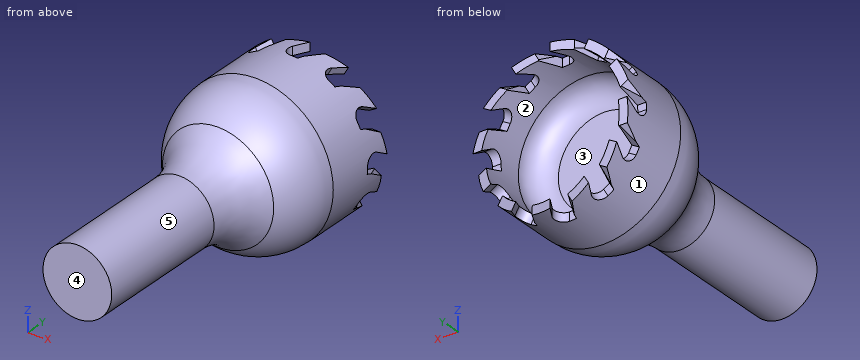
```python
from build123d import *

# Parameters (mm, degrees)
CUT_EXTRUDE1_DEPTH = 19.304
CIRPATTERN2_COUNT  = 12


with BuildPart() as part:
    # Sketch1 → Revolve1 (revolve)
    with BuildSketch(Plane.XY, mode=Mode.PRIVATE) as revolve1_sk:
        with BuildLine():
            Line((0, 0), (-4.7625, 0))
            Line((-4.7625, 0), (-4.7625, 19.05))
            ThreePointArc((-4.7625, 19.05), (-5.529894723, 22.907953795), (-7.71525, 26.178569096))
            ThreePointArc((-7.71525, 26.178569096), (-9.900605277, 29.449184398), (-10.668, 33.307138193))
            Line((-10.668, 33.307138193), (-10.668, 43.307138193))
            Line((-10.668, 43.307138193), (-9.468, 43.307138193))
            Line((-9.468, 43.307138193), (-9.468, 36.482138193))
            ThreePointArc((-9.468, 36.482138193), (-8.53806403, 34.237074162), (-6.293, 33.307138193))
            Line((-6.293, 33.307138193), (0, 33.307138193))
            Line((0, 33.307138193), (0, 0))
        make_face()
    revolve(revolve1_sk.sketch.rotate(Axis((0, 33.307138193, 0), (0, -1, 0)), 270), axis=Axis((0, 33.307138193, 0), (0, -1, 0)))

    # Sketch2 → Cut-Extrude1 (cut)
    with BuildSketch(Plane.XY):
        with BuildLine():
            Line((0, 43.307138193), (1.04608221, 41.495270656))
            ThreePointArc((1.04608221, 41.495270656), (1.04608221, 40.287358966), (0, 39.68340312))
            Line((0, 39.68340312), (-0.966946132, 39.68340312))
            Line((-0.966946132, 39.68340312), (-2.440808814, 43.792749848))
            Line((-2.440808814, 43.792749848), (4.66649361, 43.792749848))
            Line((4.66649361, 43.792749848), (4.66649361, 39.68340312))
            Line((4.66649361, 39.68340312), (2.934442802, 42.68340312))
            Line((2.934442802, 42.68340312), (0, 43.307138193))
        make_face()
    cut_extrude1 = extrude(amount=-CUT_EXTRUDE1_DEPTH, mode=Mode.SUBTRACT)

    # CirPattern2: Cut-Extrude1 ×12 about axis
    cirpattern2_axis = Axis((0, 0, 0), (0, 1, 0))
    for i in range(1, CIRPATTERN2_COUNT):
        add(cut_extrude1.rotate(cirpattern2_axis, i * 360 / CIRPATTERN2_COUNT), mode=Mode.SUBTRACT)


solid = part.part
```
The model under review builds one solid part; all positions refer to its coordinate system, in mm. Face numbers are marked on the shaded views. A direction names the side the tool comes from. Round coordinates to 2 decimals unless told otherwise and drop trailing zeros. Order: outer loops, then holes, each group sorted by start corner. A loop starts at its lowest first (then second) coordinate and runs counter-clockwise, first axis right, second up. Notation, with made-up numbers: (-2.75, 14.25) - (51.25, 14.25) arc R15 ccw to (51.25, 27.25) - close; hole circle Ø2 at (-32.5, 55.25). An arc over 180 degrees is marked (long way). Answer in a Markdown table with one row per item.
(1) Clearance check with flat-ended pins moving along their axes: P1, Ø12, axis at y = 27.5, z = 8, coming from the -X side; P2, Ø1, axis at x = 4.5, z = -8, coming from the -Y side; P3, Ø1.5, axis at x = 5.5, y = 22.5, coming from the +Z side. State where each tip first meets the part, or that it passes through.
Result set:
| item | result |
|---|---|
| P1 | stops at x = -9.92 |
| P2 | stops at y = 27.29 |
| P3 | stops at z = 2.63 |
(2) For line 1 (X direction, y = 39.5, z = 0); line 2 (X direction, y = 18, z = -0.25); line 3 (X direction, y = 36.5, z = 7.75), list the stretches that pass through material, from the lowest coordinate up. Write a range as from..to.
Result set:
| item | result |
|---|---|
| line 1 | x = -10.67..-9.47, 9.47..10.67 |
| line 2 | x = -4.76..4.76 |
| line 3 | x = -7.33..-5.44, 5.44..7.33 |
(3) Machinability: for the marked faces 1 and 2, which of the approach directions +Z, -Z, +X, -X, +Y, -Y give a long, thin tool a straight path to every point of the face, cutting with its end or side? Answer none if there is none.
Result set:
| item | result |
|---|---|
| face 1 | +Y, -Y |
| face 2 | +Y |
(4) Mouldability with a two-part tool opening along X and no side actions: class the marked faces 3, 4 and 5 as released by +X, released by -X, zero draft, split by the parting line, or undercut.
Result set:
| item | result |
|---|---|
| face 3 | undercut |
| face 4 | zero draft |
| face 5 | split by the parting line |
(5) Take a section at A-A on y = 39. Write out the cut boundary in (x, z).
Result set:
| item | result |
|---|---|
| outline | circle Ø21.34 at (0, 0); hole circle Ø18.94 at (0, 0) |
(6) Take a section at B-B on y = 15. Write out the cut boundary in (x, z) (1 decimal).
Result set:
| item | result |
|---|---|
| outline | circle Ø9.5 at (0, 0) |
